Work out the finished part from the listing and answer in its coordinate system (mm). A direction names the side the tool comes from. Give positions to 0.01 mm unless a question says otherwise; leave off trailing zeros. Loops run counter-clockwise (first coordinate to the right, second up) from the corner with the lowest first, then second, coordinate; pieces in that order, holes last. Notation, with made-up numbers: M 59.5,-5 L 98.5,-5 A28 cw 98.5,20 Z; hole C 9.25,86.25 d7. An arc over 180 degrees is marked long. Answer as a JSON object with one key per item and string values. Group by question number.
```python
from build123d import *

# Parameters (mm, degrees)
BOSS_EXTRUDE1_DEPTH                          = 4
SKETCH2_W                                    = 72
SKETCH2_H                                    = 4
BOSS_EXTRUDE2_DEPTH                          = 24
CSK_FOR_M4_COUNTERSUNK_FLAT_HEAD_SCR_2_COUNT = 2
CSK_FOR_M4_COUNTERSUNK_FLAT_HEAD_SCR_2_PITCH = 31.257513815
CSK_FOR_M4_COUNTERSUNK_FLAT_HEAD_SCR_3_COUNT = 2
CSK_FOR_M4_COUNTERSUNK_FLAT_HEAD_SCR_3_PITCH = 43.237884498
CSK_FOR_M4_COUNTERSUNK_FLAT_HEAD_SCR_4_COUNT = 2
CSK_FOR_M4_COUNTERSUNK_FLAT_HEAD_SCR_4_PITCH = 71.225221445
CSK_FOR_M4_COUNTERSUNK_FLAT_HEAD_SCR_5_COUNT = 2
CSK_FOR_M4_COUNTERSUNK_FLAT_HEAD_SCR_5_PITCH = 64
CSK_FOR_M4_COUNTERSUNK_FLAT_HEAD_SCR_6_COUNT = 2
CSK_FOR_M4_COUNTERSUNK_FLAT_HEAD_SCR_6_PITCH = 32
CSK_FOR_M4_COUNTERSUNK_FLAT_HEAD_SCR_7_COUNT = 2
CSK_FOR_M4_COUNTERSUNK_FLAT_HEAD_SCR_7_PITCH = 64
FILLET1_R                                    = 1
FILLET2_R                                    = 1


with BuildPart() as part:
    # Sketch1 → Boss-Extrude1 (new body)
    with BuildSketch(Plane.XY):
        with BuildLine():
            Line((36, -225), (36, -182.992486185))
            ThreePointArc((36, -182.992486185), (0, -186.5), (-36, -182.992486185))
            Line((-36, -182.992486185), (-36, -225))
            Line((-36, -225), (36, -225))
        make_face()
    extrude(amount=-BOSS_EXTRUDE1_DEPTH)

    # Sketch2 → Boss-Extrude2 (add)
    with BuildSketch(Plane(origin=(0, 0, -4), x_dir=(-1, 0, 0), z_dir=(0, 0, -1))):
        with Locations((0, -223)):
            Rectangle(SKETCH2_W, SKETCH2_H)
    extrude(amount=BOSS_EXTRUDE2_DEPTH)

    # Sketch7 → CSK for M4 Countersunk Flat Head Screw1 (revolve, cut)
    with BuildSketch(Plane(origin=(-32, -219.25, 0), x_dir=(0, -1, 0), z_dir=(1, 0, 0))):
        Polygon((0, 0), (0, 28), (2, 28), (2, 2.05), (3.55, 0.5), (3.55, 0), align=None)
    csk_for_m4_countersunk_flat_head_screw1 = revolve(axis=Axis((-32, -219.25, 6.35), (0, 0, -1)), mode=Mode.SUBTRACT)

    # CSK for M4 Countersunk Flat Head Scr 2: CSK for M4 Countersunk Flat Head Screw1 ×2
    with Locations(*[(0, i * CSK_FOR_M4_COUNTERSUNK_FLAT_HEAD_SCR_2_PITCH, 0) for i in range(1, CSK_FOR_M4_COUNTERSUNK_FLAT_HEAD_SCR_2_COUNT)]):
        add(csk_for_m4_countersunk_flat_head_screw1, mode=Mode.SUBTRACT)

    # CSK for M4 Countersunk Flat Head Scr 3: CSK for M4 Countersunk Flat Head Screw1 ×2
    with Locations(*[Vector(0.74009171288563, 0.6725059527751515, 0) * (i * CSK_FOR_M4_COUNTERSUNK_FLAT_HEAD_SCR_3_PITCH) for i in range(1, CSK_FOR_M4_COUNTERSUNK_FLAT_HEAD_SCR_3_COUNT)]):
        add(csk_for_m4_countersunk_flat_head_screw1, mode=Mode.SUBTRACT)

    # CSK for M4 Countersunk Flat Head Scr 4: CSK for M4 Countersunk Flat Head Screw1 ×2
    with Locations(*[Vector(0.8985581048590322, 0.4388545683847263, 0) * (i * CSK_FOR_M4_COUNTERSUNK_FLAT_HEAD_SCR_4_PITCH) for i in range(1, CSK_FOR_M4_COUNTERSUNK_FLAT_HEAD_SCR_4_COUNT)]):
        add(csk_for_m4_countersunk_flat_head_screw1, mode=Mode.SUBTRACT)

    # CSK for M4 Countersunk Flat Head Scr 5: CSK for M4 Countersunk Flat Head Screw1 ×2
    with Locations(*[(i * CSK_FOR_M4_COUNTERSUNK_FLAT_HEAD_SCR_5_PITCH, 0, 0) for i in range(1, CSK_FOR_M4_COUNTERSUNK_FLAT_HEAD_SCR_5_COUNT)]):
        add(csk_for_m4_countersunk_flat_head_screw1, mode=Mode.SUBTRACT)

    # Sketch9 → CSK for M4 Countersunk Flat Head Screw2 (revolve, cut)
    with BuildSketch(Plane(origin=(32, -225, -24), x_dir=(0, 0, -1), z_dir=(1, 0, 0))):
        Polygon((0, 0), (0, 42.007513815), (2, 42.007513815), (2, 2.05), (3.55, 0.5), (3.55, 0), align=None)
    csk_for_m4_countersunk_flat_head_screw2 = revolve(axis=Axis((32, -231.35, -24), (0, 1, 0)), mode=Mode.SUBTRACT)

    # CSK for M4 Countersunk Flat Head Scr 6: CSK for M4 Countersunk Flat Head Screw2 ×2
    with Locations(*[(-i * CSK_FOR_M4_COUNTERSUNK_FLAT_HEAD_SCR_6_PITCH, 0, 0) for i in range(1, CSK_FOR_M4_COUNTERSUNK_FLAT_HEAD_SCR_6_COUNT)]):
        add(csk_for_m4_countersunk_flat_head_screw2, mode=Mode.SUBTRACT)

    # CSK for M4 Countersunk Flat Head Scr 7: CSK for M4 Countersunk Flat Head Screw2 ×2
    with Locations(*[(-i * CSK_FOR_M4_COUNTERSUNK_FLAT_HEAD_SCR_7_PITCH, 0, 0) for i in range(1, CSK_FOR_M4_COUNTERSUNK_FLAT_HEAD_SCR_7_COUNT)]):
        add(csk_for_m4_countersunk_flat_head_screw2, mode=Mode.SUBTRACT)

    # Fillet1
    fillet1_edges = [part.edges().sort_by_distance(p)[0] for p in [
        (0, -225, 0),
    ]]
    fillet(fillet1_edges, radius=FILLET1_R)

    # Fillet2
    fillet2_edges = [part.edges().sort_by_distance(p)[0] for p in [
        (-34.484122918, -221, -4),
        (34.484122918, -221, -4),
        (0, -221, -4),
    ]]
    fillet(fillet2_edges, radius=FILLET2_R)


solid = part.part
```
Item 1: Find the intervals of material crossed by probe 1 along X at (y, z) = (-222.15, -24); probe 2 along Y at (x, z) = (0, -2.9); probe 3 along Y at (x, z) = (-32, -2.75), in increasing order. Write a range as [from, to].
Item 2: A cutting plane is placed at A-A (z = -24). Determine the outline of the cut face in (x, y), and give its area (3 significant figures).
Item 3: A cutting plane is placed at D-D (z = -11.75). Determine the outline of the cut face in (x, y), and give its area (3 significant figures).
Item 4: Given pin 1 Ø6.5 at (x, z) = (-32, -24) entering from +Y; pin 2 Ø6.5 at (x, y) = (32, -187.99) entering from +Z; pin 3 Ø3.5 at (x, z) = (32, -24) entering from -Y; pin 4 Ø5.5 at (x, z) = (0, -24) entering from -Y, each flat-ended and moving along its own axis, determine where each tip first touches the part or whether it passes through.
Item 5: A tool of negligible diameter and unlimited length cuts with its end or side. For faces 1 (the cylindrical face through (31.844, -184.446, -0.246)), 2 (the cylindrical face through (29.601, -224.754, -21.384)), 3 (the flat face through (-34, -221, -16)), from which of +Z, -Z, +X, -X, +Y, -Y can it reach the whole face along a straight path? Write none if from no direction.
Item 6: A cutting plane is placed at B-B (x = 0). Determine the outline of the cut face in (y, z), and give its area (3 significant figures).
Item 7: For a pull along X with two mould halves and no side action, classify faces 4 (the cylindrical face through (30.934, -222.636, -0.246)), 5 (the flat face through (-1, -201, -4)), 6 (the flat face through (-36, -212, -3)) as pulls with the +X half, pulls with the -X half, needs draft (parallel to the pull), parting line crosses it, or undercut.
Item 8: A cutting plane is placed at C-C (y = -219.25). Determine the outline of the cut face in (x, z).
The answers:
{
 "1": {"probe 1": "x = [-36, -34], [-30, -2], [2, 30], [34, 36]", "probe 2": "y = [-225, -192.17], [-188.17, -186.5]", "probe 3": "y = [-225, -221.25], [-217.25, -189.99], [-185.99, -183.73]"},
 "2": {"outline": "M -36,-225 L -35.55,-225 L -35.55,-224.5 L -34,-222.95 L -34,-221 L -36,-221 Z; M -30,-222.95 L -28.45,-224.5 L -28.45,-225 L -3.55,-225 L -3.55,-224.5 L -2,-222.95 L -2,-221 L -30,-221 Z; M 2,-222.95 L 3.55,-224.5 L 3.55,-225 L 28.45,-225 L 28.45,-224.5 L 30,-222.95 L 30,-221 L 2,-221 Z; M 34,-222.95 L 35.55,-224.5 L 35.55,-225 L 36,-225 L 36,-221 L 34,-221 Z", "area": "228 mm^2"},
 "3": {"outline": "M -36,-225 L 36,-225 L 36,-221 L 32.97,-221 A2 cw 31.03,-221 L -31.03,-221 A2 cw -32.97,-221 L -36,-221 Z", "area": "287 mm^2"},
 "4": {"pin 1": "stops at y = -221", "pin 2": "stops at z = -0.8", "pin 3": "passes through", "pin 4": "stops at y = -223.7"},
 "5": {"face 1": "+Z", "face 2": "-Y", "face 3": "-Z, +X, -X, +Y"},
 "6": {"outline": "M -225,-28 L -221,-28 L -221,-26 L -222.95,-26 L -224.5,-27.55 L -225,-27.55 Z; M -225,-20.45 L -224.5,-20.45 L -222.95,-22 L -221,-22 L -221,-5 A1 cw -220,-4 L -192.17,-4 L -192.17,-2.05 L -193.72,-0.5 L -193.72,0 L -224,0 A1 ccw -225,-1 Z; M -188.17,-4 L -186.5,-4 L -186.5,0 L -186.62,0 L -186.62,-0.5 L -188.17,-2.05 Z", "area": "210 mm^2"},
 "7": {"face 4": "undercut", "face 5": "needs draft", "face 6": "pulls with the -X half"},
 "8": {"outline": "M -36,-4 L -34,-4 L -34,-2.05 L -35.55,-0.5 L -35.55,0 L -36,0 Z; M -30,-4 L 30,-4 L 30,-2.05 L 28.45,-0.5 L 28.45,0 L -28.45,0 L -28.45,-0.5 L -30,-2.05 Z; M 34,-4 L 36,-4 L 36,0 L 35.55,0 L 35.55,-0.5 L 34,-2.05 Z"}
}
